```python
from build123d import *

# Parameters (mm, degrees)
CROQUIS2_W              = 120
CROQUIS2_H              = 200
SALIENTE_EXTRUIR1_DEPTH = 200
VACIADO1_T              = -3
CROQUIS4_R              = 10
SALIENTE_EXTRUIR2_DEPTH = 80


with BuildPart() as part:
    # Croquis2 → Saliente-Extruir1 (new body)
    with BuildSketch(Plane.XY):
        with Locations((60, 100)):
            Rectangle(CROQUIS2_W, CROQUIS2_H)
    extrude(amount=SALIENTE_EXTRUIR1_DEPTH)

    # Vaciado1
    vaciado1_openings = [part.faces().sort_by_distance(p)[0] for p in [
        (60, 100, 200),
    ]]
    offset(amount=VACIADO1_T, openings=vaciado1_openings, kind=Kind.INTERSECTION)

    # Croquis4 → Saliente-Extruir2 (add)
    with BuildSketch(Plane.ZY.offset(-117)):
        with Locations((100, 100)):
            Circle(CROQUIS4_R)
    extrude(amount=SALIENTE_EXTRUIR2_DEPTH)


solid = part.part
```
The model under review builds one solid part; all positions refer to its coordinate system, in mm. A direction names the side the tool comes from. Give positions to 0.01 mm unless a question says otherwise; leave off trailing zeros. Write each loop counter-clockwise with the first axis right and the second up, starting at its lowest first coordinate (ties: lowest second). Pieces come first, ordered by that corner, then holes. Notation, with made-up numbers: (52.5, 71.25) -> (96.5, 71.25) arc R25 ccw to (96.5, 100.25) -> close; hole circle Ø2 at (89.25, -15). An arc over 180 degrees is marked (long way). Put each result on its own line as item: value.
(1) Tool access review of faces 1 (the flat face through (59, 197, 100)), 2 (the flat face through (59, 200, 99)): name each direction out of +Z, -Z, +X, -X, +Y, -Y from which nothing blocks a thin tool from reaching the whole face with its end or side.
Results are:
face 1: +Z
face 2: +Z, -Z, +X, -X, +Y
(2) We need section B-B, the plane y = 180.5. Give the boundary of the cut face in (x, z).
Results are:
outline: (0, 0) -> (120, 0) -> (120, 200) -> (117, 200) -> (117, 3) -> (3, 3) -> (3, 200) -> (0, 200) -> close
(3) To check wall thickness, follow probe 1 along Y at (x, z) = (89.5, 99); probe 2 along X at (y, z) = (82, 29.5); probe 3 along Y at (x, z) = (9, 15). State the ranges of each line that lie inside material, in increasing order. Write a range as from..to.
Results are:
probe 1: 0..3, 90.05..109.95, 197..200
probe 2: 0..3, 117..120
probe 3: 0..3, 197..200
(4) We need section A-A, the plane z = 100. Give the boundary of the cut face in (x, y).
Results are:
outline: (0, 0) -> (120, 0) -> (120, 200) -> (0, 200) -> close; hole (3, 3) -> (117, 3) -> (117, 90) -> (37, 90) -> (37, 110) -> (117, 110) -> (117, 197) -> (3, 197) -> close
(5) We need section D-D, the plane y = 100. Give the boundary of the cut face in (x, z).
Results are:
outline: (0, 0) -> (120, 0) -> (120, 200) -> (117, 200) -> (117, 110) -> (37, 110) -> (37, 90) -> (117, 90) -> (117, 3) -> (3, 3) -> (3, 200) -> (0, 200) -> close
(6) For pin 1 Ø1.5 at (x, y) = (39, 57.5) entering from +Z, flat-tipped, find the tip position at first contact; note if it passes through.
Results are:
pin 1: z = 3
(7) The part is to be moulded in two halves that separate along X. For faces 3 (the flat face through (59, 3, 100)), 4 (the flat face through (2, 100, 200)), 5 (the cylindrical face through (77.56, 109.915, 98.698)), 6 (the flat face through (120, 99, 99)), say which applies: pulls with the +X half, pulls with the -X half, needs draft (parallel to the pull), parting line crosses it, or undercut.
Results are:
face 3: undercut
face 4: needs draft
face 5: undercut
face 6: pulls with the +X half
(8) We need section C-C, the plane z = 186. Give the boundary of the cut face in (x, y).
Results are:
outline: (0, 0) -> (120, 0) -> (120, 200) -> (0, 200) -> close; hole (3, 3) -> (117, 3) -> (117, 197) -> (3, 197) -> close
